from build123d import *

# Parameters (mm, degrees)
F0_W      = 10
F0_H      = 7
F1_DEPTH  = 20
F2_W      = 5
F2_H      = 16
F3_DEPTH  = 7
F4_W      = 5
F4_H      = 3
F5_DEPTH  = 7
F7_DEPTH  = 5
F9_DEPTH  = 16
F10_R     = 1.5
F11_DEPTH = 94
F12_R     = 5
F13_DEPTH = 2238


with BuildPart() as f1:
    # F0 (on Front) → F1 (new body)
    with BuildSketch(Plane.XZ):
        Rectangle(F0_W, F0_H)
    extrude(amount=F1_DEPTH)

    # F2 (on face) → F3 (cut, through all)
    with BuildSketch(Plane.XY.offset(3.5)):
        with Locations((0, -10)):
            Rectangle(F2_W, F2_H)
    extrude(amount=-F3_DEPTH, mode=Mode.SUBTRACT)

    # F4 (on face) → F5 (join, through all)
    with BuildSketch(Plane(origin=(0, 0, -3.5), x_dir=(1, 0, 0), z_dir=(0, 0, -1))):
        with Locations((0, 3.5)):
            Rectangle(F4_W, F4_H)
        with Locations((0, 16.5)):
            Rectangle(F4_W, F4_H)
    extrude(amount=-F5_DEPTH)

    # F6 (on face) → F7 (cut, through all)
    with BuildSketch(Plane(origin=(2.5, 0, 0), x_dir=(0, -1, 0), z_dir=(-1, 0, 0))):
        Polygon((2.5, 3.5), (5, 1.841688), (5, 3.5), align=None)
        Polygon((2.5, -3.5), (5, -3.5), (5, -1.841688), align=None)
        Polygon((17.5, 3.5), (15, 3.5), (15, 1.841688), align=None)
    extrude(amount=F7_DEPTH, mode=Mode.SUBTRACT)

    # F8 (on face) → F9 (join)
    with BuildSketch(Plane(origin=(0, 0, 0), x_dir=(-1, 0, 0), z_dir=(0, 1, 0))):
        with BuildLine():
            ThreePointArc((0, -3.5), (2.474874, -2.474874), (3.5, 0))
            ThreePointArc((3.5, 0), (2.474874, 2.474874), (0, 3.5))
            ThreePointArc((0, 3.5), (-3.5, 0), (0, -3.5))
        make_face()
    extrude(amount=F9_DEPTH)

    # F10 (on face) → F11 (join)
    with BuildSketch(Plane(origin=(0, 16, 0), x_dir=(-1, 0, 0), z_dir=(0, 1, 0))):
        Circle(F10_R)
    extrude(amount=F11_DEPTH)

    # F12 (on face) → F13 (join)
    with BuildSketch(Plane(origin=(0, 110, 0), x_dir=(-1, 0, 0), z_dir=(0, 1, 0))):
        Circle(F12_R)
    extrude(amount=F13_DEPTH)


solid = f1.part
For this review, take the finished solid that the model builds, in its own axes (mm). Round coordinates to 2 decimals unless told otherwise and drop trailing zeros. Write each loop counter-clockwise with the first axis right and the second up, starting at its lowest first coordinate (ties: lowest second). Pieces come first, ordered by that corner, then holes. Notation, with made-up numbers: M 62,30 L 111,30 A14 cw 111,57 Z; hole C 24.25,-27.5 d6. An arc over 180 degrees is marked long. Write item = value, one per line. Start each with the question number.
(1) Clearance check with flat-ended pins moving along their axes: pin 1 Ø1 at (x, y) = (-3.5, 1749.5) entering from -Z; pin 2 Ø5 at (y, z) = (659.5, 2) entering from +X; pin 3 Ø2 at (x, y) = (-1.5, 1937.5) entering from -Z. State where each tip first meets the part, or that it passes through.
(2) We need section A-A (y = 1142). Give the boundary of the cut face in (x, z).
(3) For line 1 along Y through (x, z) = (1.75, 1.5); line 2 along Y through (x, z) = (-0.5, 3.25); line 3 along Y through (x, z) = (-0.25, -0.25), list the stretches that pass through material, from the lowest coordinate up.
Results found:
q1.pin_1 = -4
q1.pin_2 = 5
q1.pin_3 = -4.97
q2.outline = C 0,0 d10
q3.line_1 = -20 to -15, -5 to 16, 110 to 2348
q3.line_2 = -20 to -17.12, -2.88 to 16, 110 to 2348
q3.line_3 = -20 to -15, -5 to 2348
